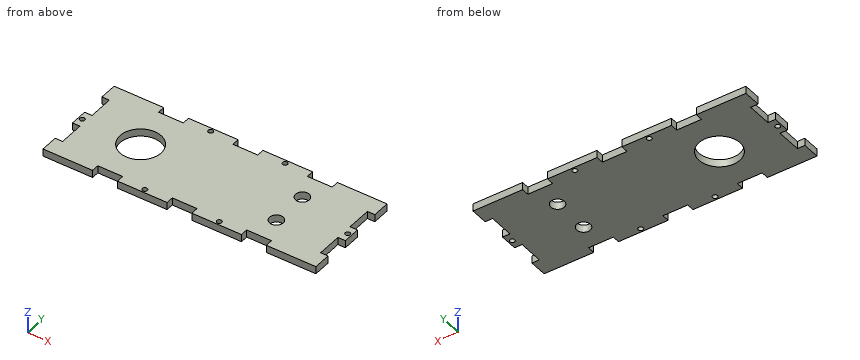
```python
from build123d import *

# Parameters (mm, degrees)
F0_R     = 1
F0_R_2   = 2.75
F0_R_3   = 8.25
F1_DEPTH = 3


with BuildPart() as f1:
    # F0 (on Top) → F1 (new body)
    with BuildSketch(Plane.XY):
        Polygon((0, 7), (0, 0), (20, 0), (20, 3), (30, 3), (30, 0), (50, 0), (50, 3), (55, 3), (60, 3), (60, 0), (80, 0), (80, 3), (90, 3), (90, 0), (110, 0), (110, 7), (107, 7), (107, 17), (110, 17), (110, 24), (107, 24), (107, 34), (110, 34), (110, 41), (90, 41), (90, 38), (80, 38), (80, 41), (60, 41), (60, 38), (55, 38), (50, 38), (50, 41), (30, 41), (30, 38), (20, 38), (20, 41), (0, 41), (0, 34), (3, 34), (3, 24), (0, 24), (0, 17), (3, 17), (3, 7), align=None)
        with Locations((40, 1.5)):
            Circle(F0_R, mode=Mode.SUBTRACT)
        with Locations((70, 1.5)):
            Circle(F0_R, mode=Mode.SUBTRACT)
        with Locations((85, 13)):
            Circle(F0_R_2, mode=Mode.SUBTRACT)
        with Locations((1.5, 20.5)):
            Circle(F0_R, mode=Mode.SUBTRACT)
        with Locations((25, 20.5)):
            Circle(F0_R_3, mode=Mode.SUBTRACT)
        with Locations((40, 39.5)):
            Circle(F0_R, mode=Mode.SUBTRACT)
        with Locations((108.5, 20.5)):
            Circle(F0_R, mode=Mode.SUBTRACT)
        with Locations((85, 28)):
            Circle(F0_R_2, mode=Mode.SUBTRACT)
        with Locations((70, 39.5)):
            Circle(F0_R, mode=Mode.SUBTRACT)
    extrude(amount=F1_DEPTH)


solid = f1.part
```
Read the model definition and answer for the solid it produces. Units are mm, in the model's axes. Coordinates: 2 decimals unless noted, no trailing zeros. Loops run counter-clockwise (first coordinate to the right, second up) from the corner with the lowest first, then second, coordinate; pieces in that order, holes last. Notation, with made-up numbers: (7.5, -35) -> (63.5, -35) arc R27 cw to (63.5, -5) -> close; hole circle Ø6 at (75, 75). An arc over 180 degrees is marked (long way). Return JSON: item names as keys, results as strings.
Item 1: Find section B-B (y = 39.5). Determine the outline of the cut face in (x, z).
Answers:
{"outline": "(0, 0) -> (20, 0) -> (20, 3) -> (0, 3) -> close; (30, 0) -> (39, 0) -> (39, 3) -> (30, 3) -> close; (41, 0) -> (50, 0) -> (50, 3) -> (41, 3) -> close; (60, 0) -> (69, 0) -> (69, 3) -> (60, 3) -> close; (71, 0) -> (80, 0) -> (80, 3) -> (71, 3) -> close; (90, 0) -> (110, 0) -> (110, 3) -> (90, 3) -> close"}
Item 2: Flat-ended cylindrical pins translate along their axes: P1, Ø1, axis at y = 25, z = 1, coming from the -X side; P2, Ø1, axis at y = 9.5, z = 0.5, coming from the +X side; P3, Ø0.9, axis at x = 54, z = 1.5, coming from the -Y side; P4, Ø1.8, axis at x = 40, y = 39.5, coming from the +Z side. Find the tip coordinate at first contact, or state that the pin passes through.
Answers:
{"P1": "stops at x = 3", "P2": "stops at x = 107", "P3": "stops at y = 3", "P4": "passes through"}
Item 3: Find section D-D (x = 108.5). Determine the outline of the cut face in (y, z), plus the area to 3 significant figures.
Answers:
{"outline": "(0, 0) -> (7, 0) -> (7, 3) -> (0, 3) -> close; (17, 0) -> (19.5, 0) -> (19.5, 3) -> (17, 3) -> close; (21.5, 0) -> (24, 0) -> (24, 3) -> (21.5, 3) -> close; (34, 0) -> (41, 0) -> (41, 3) -> (34, 3) -> close", "area": "57.0 mm2"}
Item 4: Find section A-A (x = 85). Determine the outline of the cut face in (y, z), plus the area to 3 significant figures.
Answers:
{"outline": "(3, 0) -> (10.25, 0) -> (10.25, 3) -> (3, 3) -> close; (15.75, 0) -> (25.25, 0) -> (25.25, 3) -> (15.75, 3) -> close; (30.75, 0) -> (38, 0) -> (38, 3) -> (30.75, 3) -> close", "area": "72.0 mm2"}
Item 5: Find section C-C (y = 20.5). Determine the outline of the cut face in (x, z).
Answers:
{"outline": "(0, 0) -> (0.5, 0) -> (0.5, 3) -> (0, 3) -> close; (2.5, 0) -> (16.75, 0) -> (16.75, 3) -> (2.5, 3) -> close; (33.25, 0) -> (107.5, 0) -> (107.5, 3) -> (33.25, 3) -> close; (109.5, 0) -> (110, 0) -> (110, 3) -> (109.5, 3) -> close"}
Item 6: Find the intervals of material crossed by probe 1 along Y at (x, z) = (85, 2.05); probe 2 along Y at (x, z) = (40, 1.3); probe 3 along Y at (x, z) = (1.5, 1.1), in increasing order.
Answers:
{"probe 1": "y = 3 to 10.25, 15.75 to 25.25, 30.75 to 38", "probe 2": "y = 0 to 0.5, 2.5 to 38.5, 40.5 to 41", "probe 3": "y = 0 to 7, 17 to 19.5, 21.5 to 24, 34 to 41"}
